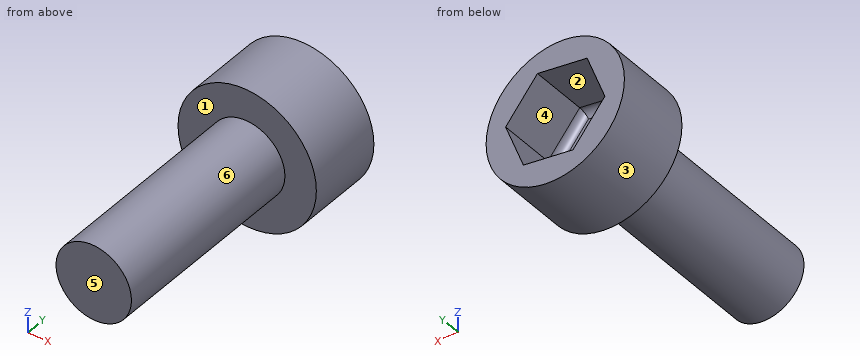
from build123d import *

# Parameters (mm, degrees)
SKETCH_1_R          = 1.5
EXTRUDE_1_DEPTH     = 8
SKETCH_2_R          = 2.75
EXTRUDE_2_DEPTH     = 3
CUT_EXTRUDE_1_DEPTH = 2.5
FILLET_1_R          = 0.3


with BuildPart() as part:
    # 草图1 → 凸台-拉伸1 (new body)
    with BuildSketch(Plane(origin=(0, 0, 0), x_dir=(1, 0, 0), z_dir=(0, 1, 0))):
        Circle(SKETCH_1_R)
    extrude(amount=EXTRUDE_1_DEPTH)

    # 草图2 → 凸台-拉伸2 (add)
    with BuildSketch(Plane(origin=(0, 8, 0), x_dir=(1, 0, 0), z_dir=(0, 1, 0))):
        Circle(SKETCH_2_R)
    extrude(amount=EXTRUDE_2_DEPTH)

    # 草图3 → 切除-拉伸1 (cut)
    with BuildSketch(Plane(origin=(0, 11, 0), x_dir=(1, 0, 0), z_dir=(0, 1, 0))):
        Polygon((1.973732301, -0.323080184), (1.266661797, 1.54776222), (-0.707070503, 1.870842405), (-1.973732301, 0.323080184), (-1.266661797, -1.54776222), (0.707070503, -1.870842405), align=None)
    extrude(amount=-CUT_EXTRUDE_1_DEPTH, mode=Mode.SUBTRACT)

    # 圆角1
    fillet_1_edges = [part.edges().sort_by_distance(p)[0] for p in [
        (1.340401402, 8.5, 1.096961295),
        (-0.279795647, 8.5, 1.709302313),
        (-1.620197049, 8.5, 0.612341018),
        (-1.340401402, 8.5, -1.096961295),
        (0.279795647, 8.5, -1.709302313),
        (1.620197049, 8.5, -0.612341018),
    ]]
    fillet(fillet_1_edges, radius=FILLET_1_R)


solid = part.part
The listing builds one solid part. Answer for the finished solid, in the listing's coordinates (mm). Face numbers are marked on the shaded views. A direction names the side the tool comes from. Coordinates: 2 decimals unless noted, no trailing zeros. Order: outer loops, then holes, each group sorted by start corner. A loop starts at its lowest first (then second) coordinate and runs counter-clockwise, first axis right, second up. Notation, with made-up numbers: M 42,-21 L 55,-21 A28 ccw 55,-3 Z; hole C 57,2.25 d6. An arc over 180 degrees is marked long. Use CSV: the item, a comma, the result in double quotes.
Q1. Straight lines are drawn through the part: L1, parallel to Y at x = 2.45, z = -1.15; L2, parallel to Y at x = -1.55, z = -0.4; L3, parallel to Z at x = -1.05, y = 10. For each, find the intervals that lie inside material, in ascending order.
Here are the results:
L1,"8 to 11"
L2,"8 to 8.5"
L3,"-2.54 to -1.45, 1.58 to 2.54"
Q2. Given pin 1 Ø3 at (x, y) = (0.5, 4.5) entering from +Z; pin 2 Ø3 at (y, z) = (5.5, 1) entering from +X; pin 3 Ø3 at (x, z) = (-1.5, 1.5) entering from -Y; pin 4 Ø1.5 at (x, z) = (-0.5, 0) entering from +Y, each flat-ended and moving along its own axis, determine where each tip first touches the part or whether it passes through.
Here are the results:
pin 1,"z = 1.5"
pin 2,"x = 1.5"
pin 3,"y = 0"
pin 4,"y = 8.5"
Q3. Section A-A (y = 9.5) is taken. Determine the outline of the cut face in (x, z), then the cut area to 3 significant figures.
Here are the results:
outline,"C 0,0 d5.5; hole M -1.97,-0.32 L -0.71,-1.87 L 1.27,-1.55 L 1.97,0.32 L 0.71,1.87 L -1.27,1.55 Z"
area,"13.4 mm2"
Q4. A tool of negligible diameter and unlimited length cuts with its end or side. For the marked faces 4, 5 and 6, from which of +Z, -Z, +X, -X, +Y, -Y can it reach the whole face along a straight path? Write none if from no direction.
Here are the results:
face 4,"+Y"
face 5,"+Z, -Z, +X, -X, -Y"
face 6,"-Y"
Q5. Section B-B (y = 6.75) is taken. Determine the outline of the cut face in (x, z).
Here are the results:
outline,"C 0,0 d3"
Q6. Determine the mould class of the marked faces 1, 2 and 3 for opening direction Z: pulls with the +Z half, pulls with the -Z half, needs draft (parallel to the pull), parting line crosses it, or undercut.
Here are the results:
face 1,"needs draft"
face 2,"undercut"
face 3,"parting line crosses it"
Q7. Section C-C (x = -2.2) is taken. Determine the outline of the cut face in (y, z), then the cut area to 3 significant figures.
Here are the results:
outline,"M 8,-1.65 L 11,-1.65 L 11,1.65 L 8,1.65 Z"
area,"9.90 mm2"
